The figure shows three views and two pictorial views of one solid part (mm, origin at its lowest corner). Answer the questions. Round coordinates to 2 decimals unless told otherwise and drop trailing zeros. Order: outer loops, then holes, each group sorted by start corner. A loop starts at its lowest first (then second) coordinate and runs counter-clockwise, first axis right, second up. Notation, with made-up numbers: (63.25, 9) -> (75.25, 9) arc R26 cw to (75.25, 36) -> close; hole circle Ø11 at (84.5, -5). An arc over 180 degrees is marked (long way). One line per item, written item: value. Start each with the question number.
1. Flat-ended cylindrical pins translate along their axes: pin 1 Ø2 at (x, y) = (54.5, 2.5) entering from -Z; pin 2 Ø2 at (y, z) = (2, 41) entering from +X; pin 3 Ø1.4 at (x, y) = (175, 2.5) entering from -Z. Find the tip coordinate at first contact, or state that the pin passes through.
2. Consider line 1 (X direction, y = 4.35, z = 36); line 2 (X direction, y = 4.1, z = 110); line 3 (Z direction, x = 53, y = 2.4). Determine where each line is inside the solid, lowest interval first.
3. Section A-A (z = 120) is taken. Give the vertices of the cut face in (x, y), then the cut area to 3 significant figures.
4. Section C-C (x = 85) is taken. Give the vertices of the cut face in (y, z).
5. Section B-B (x = 58.5) is taken. Give the vertices of the cut face in (y, z).
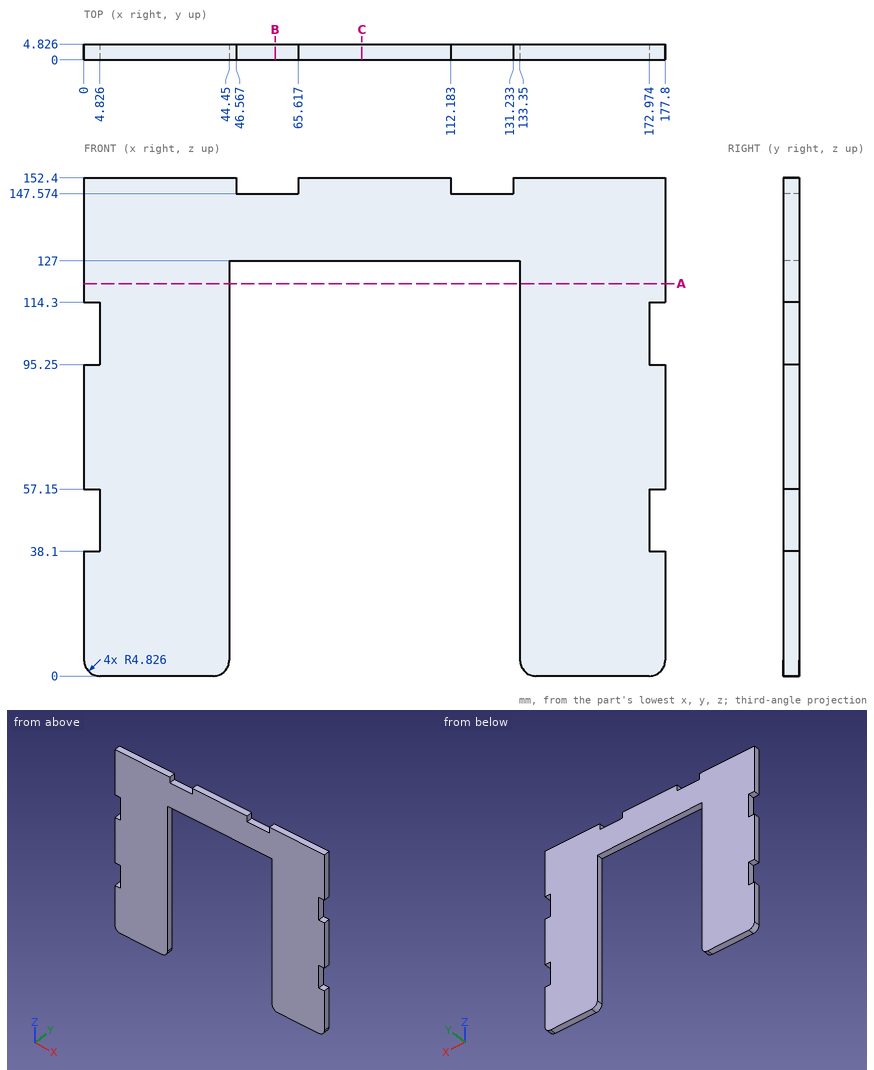
Answer:
1. pin 1: z = 127
1. pin 2: x = 172.97
1. pin 3: z = 0.19
2. line 1: 0 to 44.45, 133.35 to 177.8
2. line 2: 4.83 to 44.45, 133.35 to 172.97
2. line 3: 127 to 147.57
3. outline: (0, 0) -> (44.45, 0) -> (44.45, 4.83) -> (0, 4.83) -> close; (133.35, 0) -> (177.8, 0) -> (177.8, 4.83) -> (133.35, 4.83) -> close
3. area: 429 mm^2
4. outline: (0, 127) -> (4.83, 127) -> (4.83, 152.4) -> (0, 152.4) -> close
5. outline: (0, 127) -> (4.83, 127) -> (4.83, 147.57) -> (0, 147.57) -> close
